from build123d import *

# Parameters (mm, degrees)
BOSS_EXTRUDE1_DEPTH = 2.54
SKETCH2_R           = 2.075
CUT_EXTRUDE1_DEPTH  = 10
FILLET1_R           = 2


with BuildPart() as part:
    # Sketch1 → Boss-Extrude1 (new body)
    with BuildSketch(Plane.XY):
        with BuildLine():
            Line((52, -74), (52, 59.75))
            Line((52, 59.75), (56.25, 59.75))
            ThreePointArc((56.25, 59.75), (60.5, 64), (56.25, 68.25))
            Line((56.25, 68.25), (52, 68.25))
            Line((52, 68.25), (52, 74))
            ThreePointArc((52, 74), (51.121320344, 76.121320344), (49, 77))
            Line((49, 77), (-49, 77))
            ThreePointArc((-49, 77), (-51.121320344, 76.121320344), (-52, 74))
            Line((-52, 74), (-52, -59.75))
            Line((-52, -59.75), (-56.25, -59.75))
            ThreePointArc((-56.25, -59.75), (-60.5, -64), (-56.25, -68.25))
            Line((-56.25, -68.25), (-52, -68.25))
            Line((-52, -68.25), (-52, -74))
            ThreePointArc((-52, -74), (-51.121320344, -76.121320344), (-49, -77))
            Line((-49, -77), (49, -77))
            ThreePointArc((49, -77), (51.121320344, -76.121320344), (52, -74))
        make_face()
    extrude(amount=BOSS_EXTRUDE1_DEPTH)

    # Sketch2 → Cut-Extrude1 (cut)
    with BuildSketch(Plane.XY.offset(2.54)):
        with Locations((56.25, 64)):
            Circle(SKETCH2_R)
        with Locations((-56.25, -64)):
            Circle(SKETCH2_R)
    extrude(amount=-CUT_EXTRUDE1_DEPTH, mode=Mode.SUBTRACT)

    # Fillet1
    fillet1_edges = [part.edges().sort_by_distance(p)[0] for p in [
        (-52, -68.25, 1.27),
        (-52, -59.75, 1.27),
        (52, 68.25, 1.27),
        (52, 59.75, 1.27),
    ]]
    fillet(fillet1_edges, radius=FILLET1_R)


solid = part.part
Read the model definition and answer for the solid it produces. Units are mm, in the model's axes. Round coordinates to 2 decimals unless told otherwise and drop trailing zeros. Write each loop counter-clockwise with the first axis right and the second up, starting at its lowest first coordinate (ties: lowest second). Pieces come first, ordered by that corner, then holes.
1. The part is cut by section A-A, the plane y = 64. Determine the outline of the cut face in (x, z) (3 decimals), then the cut area to 3 significant figures.
2. The part is cut by section C-C, the plane y = 23.5. Determine the outline of the cut face in (x, z), then the cut area to 3 significant figures.
3. Determine the mould class of faces 1 (the face through (-51.1, 76.14, 1.25)), 2 (the face through (-60.5, -63.9, 1.3)), 3 (the face through (-57.9, -65.26, 1.29)) for opening direction Y: pulls with the +Y half, pulls with the -Y half, needs draft (parallel to the pull), parting line crosses it, or undercut.
4. The part is cut by section B-B, the plane z = 1.7. Determine the outline of the cut face in (x, y) (3 decimals), then the cut area to 3 significant figures.
5. Straight lines are drawn through the part: L1, parallel to Y at x = 56.25, z = 1 (3 decimals); L2, parallel to X at y = 24, z = 1.8; L3, parallel to X at y = -65, z = 1.5. For each, find the intervals that lie inside material, in ascending order.
Values:
1. outline: (-52, 0) - (54.175, 0) - (54.175, 2.54) - (-52, 2.54) - close; (58.325, 0) - (60.5, 0) - (60.5, 2.54) - (58.325, 2.54) - close
1. area: 275 mm2
2. outline: (-52, 0) - (52, 0) - (52, 2.54) - (-52, 2.54) - close
2. area: 264 mm2
3. face 1: pulls with the +Y half
3. face 2: parting line crosses it
3. face 3: undercut
4. outline: (-56.25, -68.25) - (-54, -68.25) arc R2 cw to (-52, -70.25) - (-52, -74) arc R3 ccw to (-49, -77) - (49, -77) arc R3 ccw to (52, -74) - (52, 57.75) arc R2 cw to (54, 59.75) - (56.25, 59.75) arc R4.25 ccw to (56.25, 68.25) - (54, 68.25) arc R2 cw to (52, 70.25) - (52, 74) arc R3 ccw to (49, 77) - (-49, 77) arc R3 ccw to (-52, 74) - (-52, -57.75) arc R2 cw to (-54, -59.75) - (-56.25, -59.75) arc R4.25 ccw to start; hole circle Ø4.15 at (-56.25, -64); hole circle Ø4.15 at (56.25, 64)
4. area: 16,100 mm2
5. L1: y = 59.75 to 61.925, 66.075 to 68.25
5. L2: x = -52 to 52
5. L3: x = -60.38 to -58.07, -54.43 to 52
